Geometry: see drawing. Coordinates: mm, zero at the bounding-box minimum. Give positions to 0.01 mm unless a question says otherwise; leave off trailing zeros. Write each loop counter-clockwise with the first axis right and the second up, starting at its lowest first coordinate (ties: lowest second). Pieces come first, ordered by that corner, then holes. Notation, with made-up numbers: (-24.5, -27) - (3.5, -27) arc R17 cw to (3.5, -21) - close; hole circle Ø9 at (79, 80). An arc over 180 degrees is marked (long way). One line per question, with ' | ' between items. Start each with the question number.
(1) Ray query, line 1 (Y direction, x = 18, z = 3.25); line 2 (Y direction, x = 18.5, z = 4.65); line 3 (Y direction, x = 21.5, z = 1.75). Return the intervals inside material, ascending. Write a range as [from, to].
(2) Section C-C, the plane z = 2.45. Return loops of the section in (x, y).
(3) Draft query along Y for the marked faces 1, 2 and 3. Return one class per face: +Y half, -Y half, draft (parallel to the pull), parting line (faces both ways), or undercut.
(4) Section B-B, the plane y = 32. Return loops of the section in (x, z).
(5) Section D-D, the plane x = 31. Return loops of the section in (y, z), plus the area to 3 significant figures.
(6) Section A-A, the plane x = 18. Return loops of the section in (y, z).
(7) Pin query (flat end, axial travel): pin 1 (4 mm diameter, centred on x = 16.5, y = 10, fed in from -Z); pin 2 (2 mm diameter, centred on y = 14, z = 3.5, fed in from -X); pin 3 (1.8 mm diameter, centred on x = 18, y = 32, fed in from -Z); pin 4 (1.5 mm diameter, centred on y = 7.5, z = 1, fed in from -X). Return the tip coordinate at first contact, or that it passes through.
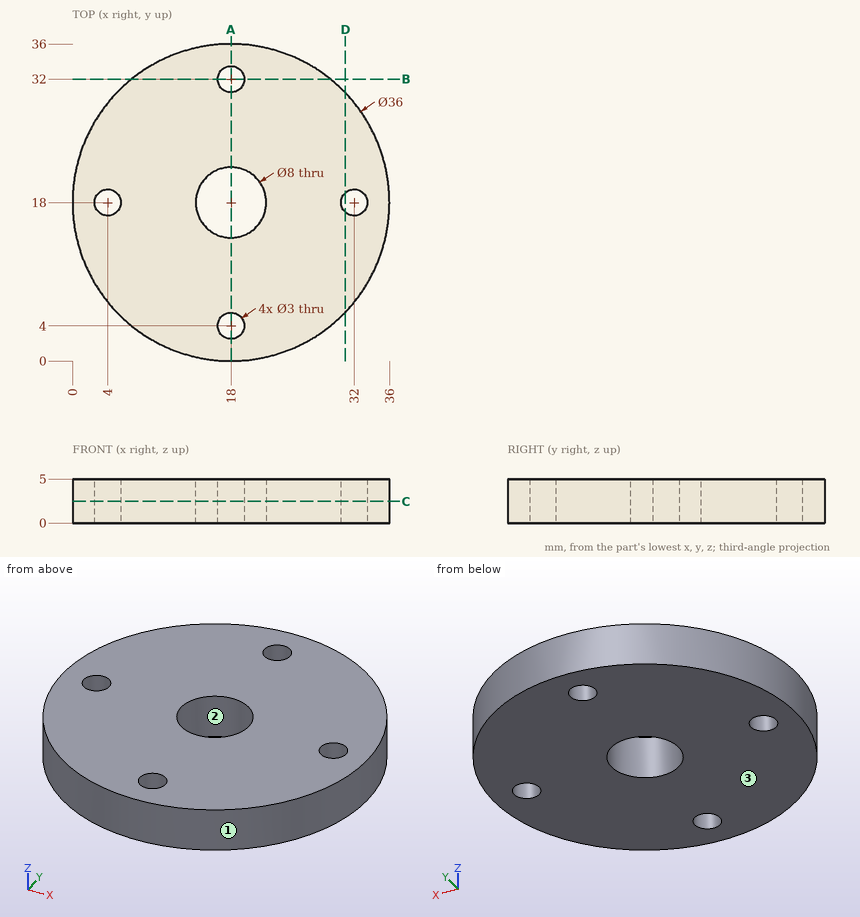
Check sheet entries:
1) line 1: [0, 2.5], [5.5, 14], [22, 30.5], [33.5, 36] | line 2: [0.01, 2.59], [5.41, 14.03], [21.97, 30.59], [33.41, 35.99] | line 3: [0.34, 16.06], [19.94, 35.66]
2) outline: circle Ø36 at (18, 18); hole circle Ø3 at (4, 18); hole circle Ø8 at (18, 18); hole circle Ø3 at (18, 4); hole circle Ø3 at (18, 32); hole circle Ø3 at (32, 18)
3) face 1: parting line | face 2: undercut | face 3: draft
4) outline: (6.69, 0) - (16.5, 0) - (16.5, 5) - (6.69, 5) - close; (19.5, 0) - (29.31, 0) - (29.31, 5) - (19.5, 5) - close
5) outline: (5.55, 0) - (16.88, 0) - (16.88, 5) - (5.55, 5) - close; (19.12, 0) - (30.45, 0) - (30.45, 5) - (19.12, 5) - close | area: 113 mm²
6) outline: (0, 0) - (2.5, 0) - (2.5, 5) - (0, 5) - close; (5.5, 0) - (14, 0) - (14, 5) - (5.5, 5) - close; (22, 0) - (30.5, 0) - (30.5, 5) - (22, 5) - close; (33.5, 0) - (36, 0) - (36, 5) - (33.5, 5) - close
7) pin 1: z = 0 | pin 2: x = 0.25 | pin 3: through | pin 4: x = 2.87
